Geometry: final body of the model. Coordinates: model frame, mm. A direction names the side the tool comes from. Give positions to 0.01 mm unless a question says otherwise; leave off trailing zeros. Order: outer loops, then holes, each group sorted by start corner. A loop starts at its lowest first (then second) coordinate and runs counter-clockwise, first axis right, second up. Notation, with made-up numbers: (41, 39) -> (66, 39) arc R20 cw to (66, 50) -> close; hole circle Ø8 at (0, -23). An arc over 180 degrees is marked (long way). Answer in a Markdown table with one row per item. Add a question column.
Q1. Cut plane A-A on y = 6. Return the cut outline in (x, z).
Q2. Pull-direction query (Z, two-part tool) for faces 1 (the face through (74, 10, -13)), 2 (the face through (10, 5, -12)), 3 (the face through (5, 5, 0)), 4 (the face through (78, 5, 3)); classes: +Z half, -Z half, draft (parallel to the pull), parting line (faces both ways), or undercut.
Q3. Set-up query: faces 5 (the face through (113, 5, -25)), 6 (the face through (5, 5, -25)), 7 (the face through (113, 5, 0)). Return all of +Z, -Z, +X, -X, +Y, -Y with unobstructed straight access to the full face (end or side cutting, diameter ignored); none if empty.
Q4. Cut plane B-B on x = 123. Return the cut outline in (y, z), and give its area (3 significant figures).
Q5. Line query: line 1 along X through (y, z) = (5.25, -12.5); line 2 along Z through (x, y) = (42, 4); line 3 along Z through (x, y) = (97, 6.25). Output: solid intervals per line, ascending. Write a range as from..to.
Q6. Cut plane C-C on z = -19.5. Return the cut outline in (x, y), and give its area (3 significant figures).
Q7. Contact query for flat-ended pins moving along their axis: P1, Ø3, axis at x = 117, y = 7, coming from the +Z side; P2, Ø3, axis at x = 97.5, y = 3.5, coming from the -Z side; P3, Ø8, axis at x = 69, z = -2.5, coming from the -Y side; P4, Ø5, axis at y = 4.5, z = -15.5, coming from the -X side. Output: stop coordinate, or through.
from build123d import *

# Parameters (mm, degrees)
EXTRUDE_1_DEPTH        = 10
SKETCH_2_R             = 0.75
CUT_EXTRUDE_1_DEPTH    = 149.613592918
PATTERN_LINEAR_1_COUNT = 2
PATTERN_LINEAR_1_PITCH = 55


with BuildPart() as part:
    # Эскиз1 → Бобышка-Вытянуть1 (new body)
    with BuildSketch(Plane(origin=(0, 0, 0), x_dir=(1, 0, 0), z_dir=(0, 1, 0))):
        Polygon((0, 31), (75, 31), (81, 25), (145, 25), (145, 0), (81, 0), (75, -6), (0, -6), (0, 0), (10, 0), (10, 25), (0, 25), align=None)
    extrude(amount=EXTRUDE_1_DEPTH)

    # Эскиз2 → Вырез-Вытянуть1 (cut, through all)
    with BuildSketch(Plane(origin=(0, 10, 0), x_dir=(1, 0, 0), z_dir=(0, 1, 0))):
        with Locations(Location((42, 12.5, 0), (0, 0, 270))):
            Circle(SKETCH_2_R)
    cut_extrude_1 = extrude(amount=-CUT_EXTRUDE_1_DEPTH, mode=Mode.SUBTRACT)

    # Линейный массив1: Вырез-Вытянуть1 ×2
    with Locations(*[(i * PATTERN_LINEAR_1_PITCH, 0, 0) for i in range(1, PATTERN_LINEAR_1_COUNT)]):
        add(cut_extrude_1, mode=Mode.SUBTRACT)


solid = part.part
Completed:
| question | item | result |
|---|---|---|
| 1 | outline | (0, -31) -> (75, -31) -> (81, -25) -> (145, -25) -> (145, 0) -> (81, 0) -> (75, 6) -> (0, 6) -> (0, 0) -> (10, 0) -> (10, -25) -> (0, -25) -> close; hole circle Ø1.5 at (42, -12.5); hole circle Ø1.5 at (97, -12.5) |
| 2 | face 1 | draft |
| 2 | face 2 | undercut |
| 2 | face 3 | undercut |
| 2 | face 4 | +Z half |
| 3 | face 5 | -Z, +X, +Y, -Y |
| 3 | face 6 | -X, +Y, -Y |
| 3 | face 7 | +Z, +X, +Y, -Y |
| 4 | outline | (0, -25) -> (10, -25) -> (10, 0) -> (0, 0) -> close |
| 4 | area | 250 mm² |
| 5 | line 1 | x = 10..41.25, 42.75..96.25, 97.75..145 |
| 5 | line 2 | z = -31..-13.25, -11.75..6 |
| 5 | line 3 | z = -25..-13.25, -11.75..0 |
| 6 | outline | (10, 0) -> (145, 0) -> (145, 10) -> (10, 10) -> close |
| 6 | area | 1,350 mm² |
| 7 | P1 | stops at z = 0 |
| 7 | P2 | stops at z = -25 |
| 7 | P3 | stops at y = 0 |
| 7 | P4 | stops at x = 10 |
